The listing builds one solid part. Answer for the finished solid, in the listing's coordinates (mm). A direction names the side the tool comes from. Coordinates: 2 decimals unless noted, no trailing zeros. Order: outer loops, then holes, each group sorted by start corner. A loop starts at its lowest first (then second) coordinate and runs counter-clockwise, first axis right, second up. Notation, with made-up numbers: (18, 66) -> (66, 66) arc R11 cw to (66, 73) -> close; hole circle Ø2 at (68, 69). An arc over 180 degrees is marked (long way). One line per question, with ' | ' between items.
from build123d import *

# Parameters (mm, degrees)
SKETCH3_W           = 10
SKETCH3_H           = 6.5
BOSS_EXTRUDE2_DEPTH = 8
CUT_EXTRUDE1_START  = 2
CUT_EXTRUDE1_DEPTH  = 6
LPATTERN2_COUNT     = 7
LPATTERN2_PITCH     = 2
SKETCH4_W           = 8
SKETCH4_H           = 7.5
BOSS_EXTRUDE3_DEPTH = 5
CUT_EXTRUDE2_START  = -3
CUT_EXTRUDE2_DEPTH  = 2
SKETCH6_R           = 1.6
CUT_EXTRUDE3_DEPTH  = 10


with BuildPart() as part:
    # Sketch3 → Boss-Extrude2 (new body)
    with BuildSketch(Plane.XY):
        with Locations((5, 1.25)):
            Rectangle(SKETCH3_W, SKETCH3_H)
    extrude(amount=BOSS_EXTRUDE2_DEPTH)

    # Sketch1 → Cut-Extrude1 (cut)
    with BuildSketch(Plane.XY.offset(CUT_EXTRUDE1_START)):
        with BuildLine():
            Line((0.740175425, 0.63), (1.259824575, 0.63))
            ThreePointArc((1.259824575, 0.63), (1.358731646, 0.667228588), (1.408543109, 0.760434783))
            ThreePointArc((1.408543109, 0.760434783), (1.442388286, 0.918062154), (1.501123596, 1.068202247))
            ThreePointArc((1.501123596, 1.068202247), (1.705850588, 1.295639059), (2, 1.38))
            Line((2, 1.38), (2, 0))
            Line((2, 0), (0, 0))
            Line((0, 0), (0, 1.38))
            ThreePointArc((0, 1.38), (0.294149412, 1.295639059), (0.498876404, 1.068202247))
            ThreePointArc((0.498876404, 1.068202247), (0.557611714, 0.918062154), (0.591456891, 0.760434783))
            ThreePointArc((0.591456891, 0.760434783), (0.641268354, 0.667228588), (0.740175425, 0.63))
        make_face()
    cut_extrude1 = extrude(amount=CUT_EXTRUDE1_DEPTH, mode=Mode.SUBTRACT)

    # LPattern2: Cut-Extrude1 ×7
    with Locations(*[(i * LPATTERN2_PITCH, 0, 0) for i in range(1, LPATTERN2_COUNT)]):
        add(cut_extrude1, mode=Mode.SUBTRACT)

    # Sketch4 → Boss-Extrude3 (add)
    with BuildSketch(Plane.ZY):
        with Locations((4, -5.75)):
            Rectangle(SKETCH4_W, SKETCH4_H)
    extrude(amount=-BOSS_EXTRUDE3_DEPTH)

    # Sketch5 → Cut-Extrude2 (cut)
    with BuildSketch(Plane.ZY.offset(CUT_EXTRUDE2_START)):
        Polygon((1.25, -4.16228676), (1.25, -7.33771324), (4, -8.925426481), (6.75, -7.33771324), (6.75, -4.16228676), (4, -2.574573519), align=None)
    extrude(amount=-CUT_EXTRUDE2_DEPTH, mode=Mode.SUBTRACT)

    # Sketch6 → Cut-Extrude3 (cut)
    with BuildSketch(Plane.ZY.offset(-3)):
        with Locations((4, -5.75)):
            Circle(SKETCH6_R)
    extrude(amount=CUT_EXTRUDE3_DEPTH, mode=Mode.SUBTRACT)


solid = part.part
Item 1: For faces 1 (the face through (5, 3, 8)), 2 (the face through (5, 0, 5)), 3 (the face through (5, 4.5, 4)), 4 (the face through (5.1, 0.4, 2)), 5 (the face through (3.99, -3.36, 2.64)), determine the directions among +Z, -Z, +X, -X, +Y, -Y from which every point of the face is accessible in a straight line to the end or side of a thin tool.
Computed values:
face 1: +Z, +X, -X, +Y, -Y | face 2: +Z, +X, -X | face 3: +Z, -Z, +X, -X, +Y | face 4: +Z | face 5: +X
Item 2: Section A-A, the plane y = -5.75 is taken. Give the vertices of the cut face in (x, z), plus the area to 3 significant figures.
Computed values:
outline: (0, 0) -> (5, 0) -> (5, 1.25) -> (3, 1.25) -> (3, 2.4) -> (0, 2.4) -> close; (0, 5.6) -> (3, 5.6) -> (3, 6.75) -> (5, 6.75) -> (5, 8) -> (0, 8) -> close | area: 19.4 mm^2
Item 3: Section C-C, the plane y = -7.75 is taken. Give the vertices of the cut face in (x, z), plus the area to 3 significant figures.
Computed values:
outline: (0, 0) -> (5, 0) -> (5, 1.96) -> (3, 1.96) -> (3, 6.04) -> (5, 6.04) -> (5, 8) -> (0, 8) -> close | area: 31.9 mm^2
Item 4: Find the intervals of material crossed by L1, parallel to Y at x = 1.65, z = 4; L2, parallel to Y at x = 0.75, z = 4; L3, parallel to Z at x = 1.05, y = -5.75, in increasing order.
Computed values:
L1: y = -9.5 to -7.35, -4.15 to 0, 1.26 to 4.5 | L2: y = -9.5 to -7.35, -4.15 to 0, 0.63 to 4.5 | L3: z = 0 to 2.4, 5.6 to 8
Item 5: Each of these flat-tipped pins is pushed along its axis until it touches: pin 1 Ø1.5 at (x, z) = (8.5, 6) entering from -Y; pin 2 Ø1.6 at (y, z) = (-7, 3.5) entering from +X. Where does it stop, or does it pass through?
Computed values:
pin 1: stops at y = -2 | pin 2: stops at x = 3
Item 6: Section D-D, the plane z = 4.5 is taken. Count the separate pieces of the cut face and the enclosed holes in it, plus the area to 3 significant figures.
Computed values:
separate pieces: 3 | enclosed holes: 0 | area: 71.9 mm^2
Item 7: Section B-B, the plane x = 3.75 is taken. Give the vertices of the cut face in (y, z), plus the area to 3 significant figures.
Computed values:
outline: (-9.5, 0) -> (4.5, 0) -> (4.5, 8) -> (1.32, 8) -> (1.32, 2) -> (0, 2) -> (0, 8) -> (-9.5, 8) -> close; hole (-8.93, 4) -> (-7.34, 1.25) -> (-4.16, 1.25) -> (-2.57, 4) -> (-4.16, 6.75) -> (-7.34, 6.75) -> close | area: 77.9 mm^2
Item 8: Determine the mould class of faces 6 (the face through (5, -3, 2)), 7 (the face through (4, -1, 0)), 8 (the face through (3.99, -8.14, 5.36)), 9 (the face through (4, -4, 8)) for opening direction Z: pulls with the +Z half, pulls with the -Z half, needs draft (parallel to the pull), parting line crosses it, or undercut.
Computed values:
face 6: needs draft | face 7: pulls with the -Z half | face 8: undercut | face 9: pulls with the +Z half
